Can you work these out from the model? Positions are in its coordinate system, mm. A direction names the side the tool comes from. Coordinates: 2 decimals unless noted, no trailing zeros. Loops run counter-clockwise (first coordinate to the right, second up) from the corner with the lowest first, then second, coordinate; pieces in that order, holes last. Notation, with made-up numbers: (-39, 44) - (-15, 44) arc R3 ccw to (-15, 48) - close; hole circle Ø6 at (54.5, 71.5). An arc over 180 degrees is marked (long way). Put each result on its own line as item: value. Start each with the question number.
from build123d import *

# Parameters (mm, degrees)
BOSS_EXTRUDE2_DEPTH = 9
SKETCH6_R           = 1.75
SKETCH6_W           = 7
SKETCH6_H           = 5.1
CUT_EXTRUDE1_DEPTH  = 8


with BuildPart() as part:
    # Sketch4 → Boss-Extrude2 (new body)
    with BuildSketch(Plane(origin=(0, 0, 0), x_dir=(0, 0, -1), z_dir=(1, 0, 0))):
        Polygon((0, 0), (0, -4), (-7, -4), (-7, 3), (7, 3), (7, 0), align=None)
    extrude(amount=BOSS_EXTRUDE2_DEPTH)

    # Sketch6 → Cut-Extrude1 (cut, through all)
    with BuildSketch(Plane(origin=(0, 3, 0), x_dir=(1, 0, 0), z_dir=(0, 1, 0))):
        with Locations((4.5, 4)):
            Circle(SKETCH6_R)
        with Locations((4.5, -3.5)):
            Rectangle(SKETCH6_W, SKETCH6_H)
    extrude(amount=-CUT_EXTRUDE1_DEPTH, mode=Mode.SUBTRACT)


solid = part.part
Q1. Please list where these lines run through material, in increasing order: line 1 along Z through (x, y) = (4.5, 1.05); line 2 along X through (y, z) = (-2.25, 3.5); line 3 along X through (y, z) = (2, -4). Write a range as [from, to].
Q2. On a 3-axis mill with a long thin cutter (end or side, diameter ignored), from which of +Z, -Z, +X, -X, +Y, -Y can I reach the whole of each face in a straight line? I mean faces 4 (the flat face through (4, 3, -1)), 5 (the flat face through (4, 0, -2)), 6 (the flat face through (1, 0, 4)). Say none if no direction works.
Q3. I want a section at B-B on x = 4.5. List the corners of the cut face in (y, z) for me.
Q4. I want a section at C-C on y = 2.5. List the corners of the cut face in (x, z) for me.
Q5. I want a section at D-D on x = 7.5. List the corners of the cut face in (y, z) for me.
Q6. Will this pin go through, and if not, where does the flat tip stop? pin 1 (4.5 mm diameter, centred on x = 4.5, z = -4, fed in from -Y).
Q7. I want a section at A-A on z = 2.5. List the corners of the cut face in (x, y) for me.
Q8. We'd pull the mould along X, two halves only. Please class faces 1 (the flat face through (4, 2, -7)), 2 (the flat face through (9, 0, 1)), 3 (the flat face through (8, 0, 4)): released by +X, released by -X, zero draft, split by the parting line, or undercut.
Calculated:
1. line 1: [-7, -5.75], [-2.25, 0.95], [6.05, 7]
1. line 2: [0, 1], [8, 9]
1. line 3: [0, 2.75], [6.25, 9]
2. face 4: +Z, -Z, +X, -X, +Y
2. face 5: -Z, +X, -X, -Y
2. face 6: +Y, -Y
3. outline: (-4, 0) - (0, 0) - (0, -2.25) - (3, -2.25) - (3, 0.95) - (-4, 0.95) - close; (-4, 6.05) - (3, 6.05) - (3, 7) - (-4, 7) - close; (0, -7) - (3, -7) - (3, -5.75) - (0, -5.75) - close
4. outline: (0, -7) - (9, -7) - (9, 7) - (0, 7) - close; hole (1, 0.95) - (8, 0.95) - (8, 6.05) - (1, 6.05) - close; hole circle Ø3.5 at (4.5, -4)
5. outline: (-4, 0) - (0, 0) - (0, -7) - (3, -7) - (3, 0.95) - (-4, 0.95) - close; (-4, 6.05) - (3, 6.05) - (3, 7) - (-4, 7) - close
6. pin 1: y = 0
7. outline: (0, -4) - (1, -4) - (1, 3) - (0, 3) - close; (8, -4) - (9, -4) - (9, 3) - (8, 3) - close
8. face 1: zero draft
8. face 2: released by +X
8. face 3: undercut
